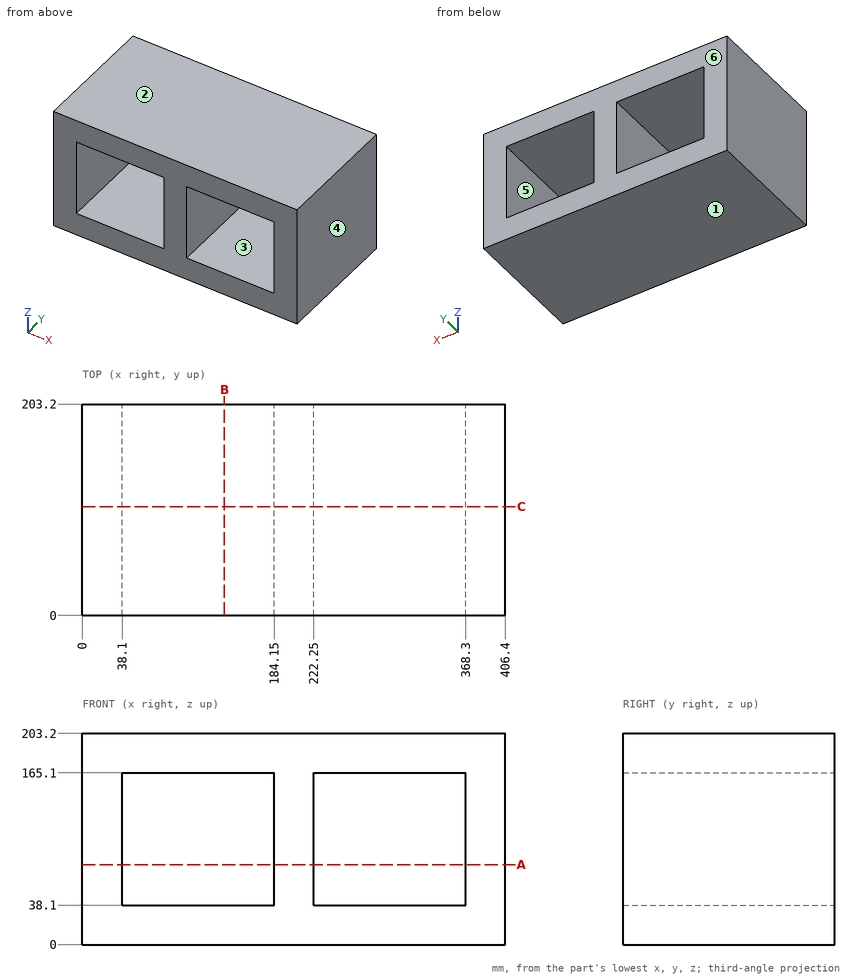
Part print with two shaded views. Sizes in mm from the minimum x, y, z corner. A direction names the side the tool comes from. Round coordinates to 2 decimals unless told otherwise and drop trailing zeros. Loops run counter-clockwise (first coordinate to the right, second up) from the corner with the lowest first, then second, coordinate; pieces in that order, holes last.
Item 1: Saw through at A-A (z = 77). List the corners of the cut face in (x, y).
Item 2: Two-plate mould, pull along Z, no slides. Class the marked faces 1, 2, 3 and 4: released by +Z, released by -Z, zero draft, split by the parting line, or undercut.
Item 3: Drill centre lines: line 1 along X through (y, z) = (40.5, 108); line 2 along Z through (x, y) = (146.5, 101). Where is each one in solid material? Low to high.
Item 4: Saw through at B-B (x = 136.5). List the corners of the cut face in (y, z), then the cut area to 3 significant figures.
Item 5: Which spindle directions (+Z, -Z, +X, -X, +Y, -Y) get a long thin tool onto all of the face, cutting with end or side? Do the marked faces 5 and 6. Say none if no direction does.
Item 6: Saw through at C-C (y = 104.5). List the corners of the cut face in (x, z), then the cut area to 3 significant figures.
Worked answers:
1. outline: (0, 0) - (38.1, 0) - (38.1, 203.2) - (0, 203.2) - close; (184.15, 0) - (222.25, 0) - (222.25, 203.2) - (184.15, 203.2) - close; (368.3, 0) - (406.4, 0) - (406.4, 203.2) - (368.3, 203.2) - close
2. face 1: released by -Z
2. face 2: released by +Z
2. face 3: undercut
2. face 4: zero draft
3. line 1: x = 0 to 38.1, 184.15 to 222.25, 368.3 to 406.4
3. line 2: z = 0 to 38.1, 165.1 to 203.2
4. outline: (0, 0) - (203.2, 0) - (203.2, 38.1) - (0, 38.1) - close; (0, 165.1) - (203.2, 165.1) - (203.2, 203.2) - (0, 203.2) - close
4. area: 15,500 mm2
5. face 5: +Y, -Y
5. face 6: +Z, -Z, +X, -X, +Y
6. outline: (0, 0) - (406.4, 0) - (406.4, 203.2) - (0, 203.2) - close; hole (38.1, 38.1) - (184.15, 38.1) - (184.15, 165.1) - (38.1, 165.1) - close; hole (222.25, 38.1) - (368.3, 38.1) - (368.3, 165.1) - (222.25, 165.1) - close
6. area: 45,500 mm2
